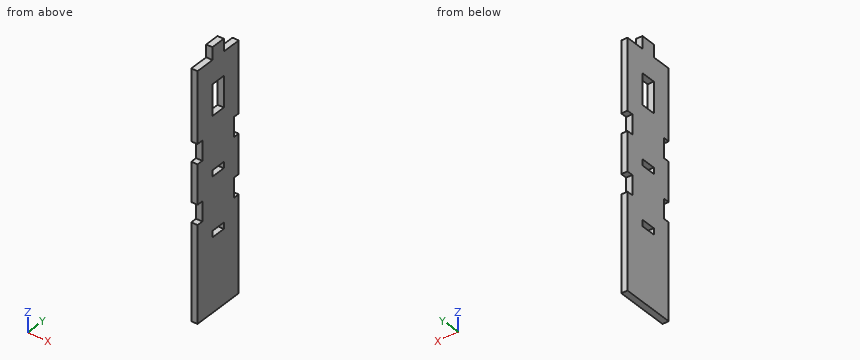
```python
from build123d import *

# Parameters (mm, degrees)
SKETCH1_W           = 250
SKETCH1_H           = 54.7
SKETCH1_W_2         = 12.7
SKETCH1_H_2         = 15
BOSS_EXTRUDE1_DEPTH = 6.35
SKETCH2_W           = 6.35
SKETCH2_H           = 15
CUT_EXTRUDE1_DEPTH  = 141.533394608
LPATTERN1_COUNT     = 3
LPATTERN1_PITCH     = 60
SKETCH3_W           = 25
SKETCH3_H           = 15
CUT_EXTRUDE2_DEPTH  = 141.533394608
SKETCH4_W           = 20
SKETCH4_H           = 6.35
CUT_EXTRUDE3_DEPTH  = 141.533394608


with BuildPart() as part:
    # Sketch1 → Boss-Extrude1 (new body)
    with BuildSketch(Plane(origin=(0, 0, 0), x_dir=(0, 0, -1), z_dir=(1, 0, 0))):
        Rectangle(SKETCH1_W, SKETCH1_H)
        with Locations((-131.35, 0)):
            Rectangle(SKETCH1_W_2, SKETCH1_H_2)
    extrude(amount=BOSS_EXTRUDE1_DEPTH)

    # Sketch2 → Cut-Extrude1 (cut, through all)
    with BuildSketch(Plane(origin=(6.35, 0, 0), x_dir=(0, 0, -1), z_dir=(1, 0, 0))):
        with Locations((-72.825, 0)):
            Rectangle(SKETCH2_W, SKETCH2_H)
    cut_extrude1 = extrude(amount=-CUT_EXTRUDE1_DEPTH, mode=Mode.SUBTRACT)

    # LPattern1: Cut-Extrude1 ×3
    with Locations(*[(0, 0, -i * LPATTERN1_PITCH) for i in range(1, LPATTERN1_COUNT)]):
        add(cut_extrude1, mode=Mode.SUBTRACT)

    # Sketch3 → Cut-Extrude2 (cut, through all)
    with BuildSketch(Plane(origin=(6.35, 0, 0), x_dir=(0, 0, -1), z_dir=(1, 0, 0))):
        with Locations((-88.5, 0)):
            Rectangle(SKETCH3_W, SKETCH3_H)
    extrude(amount=-CUT_EXTRUDE2_DEPTH, mode=Mode.SUBTRACT)

    # Sketch4 → Cut-Extrude3 (cut, through all)
    with BuildSketch(Plane(origin=(6.35, 0, 0), x_dir=(0, 0, -1), z_dir=(1, 0, 0))):
        with Locations((-42.825, 24.175)):
            Rectangle(SKETCH4_W, SKETCH4_H)
        with Locations((17.175, 24.175)):
            Rectangle(SKETCH4_W, SKETCH4_H)
    cut_extrude3 = extrude(amount=-CUT_EXTRUDE3_DEPTH, mode=Mode.SUBTRACT)

    # Mirror1: Cut-Extrude3 across plane
    add(cut_extrude3.mirror(Plane.ZX), mode=Mode.SUBTRACT)


solid = part.part
```
The listing builds one solid part. Answer for the finished solid, in the listing's coordinates (mm). Round coordinates to 2 decimals unless told otherwise and drop trailing zeros. Order: outer loops, then holes, each group sorted by start corner. A loop starts at its lowest first (then second) coordinate and runs counter-clockwise, first axis right, second up. Notation, with made-up numbers: (80, -35) - (96, -35) arc R33 cw to (96, -3) - close; hole circle Ø8 at (36, 22). An arc over 180 degrees is marked (long way). Put each result on its own line as item: value. Start each with the question number.
(1) Find section C-C (x = 2.5). State how many separate pieces and enclosed holes the cut face has, plus the area to 3 significant figures.
(2) Find section B-B (y = 0). Give the vertices of the cut face in (x, z), plus the area to 3 significant figures.
(3) Find section D-D (y = -14). Give the vertices of the cut face in (x, z).
(4) Given P1, Ø1.9, axis at x = 3, y = -16, coming from the +Z side; P2, Ø1.9, axis at x = 4, z = 131.5, coming from the +Y side; P3, Ø1.9, axis at x = 2.5, z = -16.5, coming from the +Y side, each flat-ended and moving along its own axis, determine where each tip first touches the part or whether it passes through.
(5) Straight lines are drawn through the part: probe 1 along Z at (x, y) = (3.5, 3); probe 2 along Z at (x, y) = (0.5, 25.5) (3 decimals); probe 3 along Y at (x, z) = (4, -47). For each, find the intervals that lie inside material, in ascending order. Write a range as from..to.
(6) Find section A-A (z = 94). Give the vertices of the cut face in (x, y), plus the area to 3 significant figures.
Reply:
1. separate pieces: 1
1. enclosed holes: 3
1. area: 12,700 mm^2
2. outline: (0, -125) - (6.35, -125) - (6.35, -50.35) - (0, -50.35) - close; (0, -44) - (6.35, -44) - (6.35, 9.65) - (0, 9.65) - close; (0, 16) - (6.35, 16) - (6.35, 69.65) - (0, 69.65) - close; (0, 101) - (6.35, 101) - (6.35, 137.7) - (0, 137.7) - close
2. area: 1,390 mm^2
3. outline: (0, -125) - (6.35, -125) - (6.35, 125) - (0, 125) - close
4. P1: z = 125
4. P2: y = 7.5
4. P3: y = 21
5. probe 1: -125..-50.35, -44..9.65, 16..69.65, 101..137.7
5. probe 2: -125..-27.175, -7.175..32.825, 52.825..125
5. probe 3: -27.35..-7.5, 7.5..27.35
6. outline: (0, -27.35) - (6.35, -27.35) - (6.35, -7.5) - (0, -7.5) - close; (0, 7.5) - (6.35, 7.5) - (6.35, 27.35) - (0, 27.35) - close
6. area: 252 mm^2
